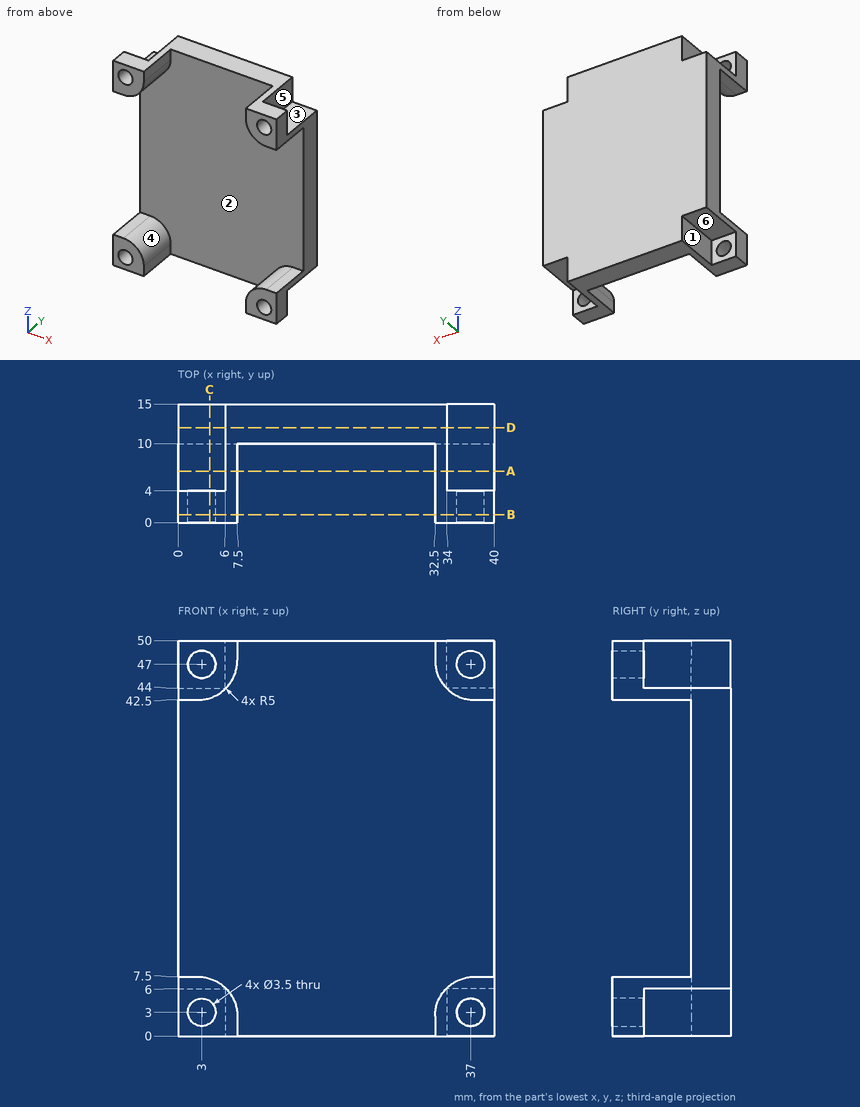
Print and shaded views of the part. All mm, measured from the part's lowest x, y and z. A direction names the side the tool comes from. Give positions to 0.01 mm unless a question says otherwise; leave off trailing zeros. Write each loop counter-clockwise with the first axis right and the second up, starting at its lowest first coordinate (ties: lowest second). Pieces come first, ordered by that corner, then holes. Notation, with made-up numbers: (62.25, 68.5) - (71.25, 68.5) arc R6 ccw to (71.25, 79.5) - close; hole circle Ø7 at (-5, 28.5). An arc over 180 degrees is marked (long way). One line per question, with ' | ' between items. Start each with the question number.
(1) Slice it at D-D on y = 12. Write the cut outline in (x, z).
(2) Wall check: line 1 along X through (y, z) = (2.5, 47); line 2 along Z through (x, y) = (37, 0.8); line 3 along Y through (x, z) = (14.5, 39.5). Give the ranges that are in metal, low to high. Write a range as from..to.
(3) Slice it at C-C on x = 4. Write the cut outline in (y, z).
(4) 3-axis set-ups, long thin cutter, end or side, ignore diameter. For the marked faces 1, 2 and 3: which of +Z, -Z, +X, -X, +Y, -Y reach the whole face in a straight line?
(5) Pin check, flat tips, straight feed: P1, Ø0.8, axis at y = 5.5, z = 0.5, coming from the -X side; P2, Ø0.8, axis at x = 2, y = 5.5, coming from the +Z side; P3, Ø4, axis at y = 7.5, z = 22, coming from the +X side; P4, Ø1.8, axis at x = 3, z = 48.5, coming from the +Y side. Stop position of each tip, or through.
(6) Two-plate mould, pull along Z, no slides. Class the marked faces 4, 5 and 6: +Z half, -Z half, draft (parallel to the pull), parting line (faces both ways), or undercut.
(7) Slice it at B-B on y = 1. Write the cut outline in (x, z).
(8) Slice it at A-A on y = 6.5. Write the cut outline in (x, z), plus the area to 3 significant figures.
Results below:
1) outline: (0, 6) - (6, 6) - (6, 0) - (34, 0) - (34, 6) - (40, 6) - (40, 44) - (34, 44) - (34, 50) - (6, 50) - (6, 44) - (0, 44) - close
2) line 1: 0..1.25, 4.75..7.47, 32.53..35.25, 38.75..40 | line 2: 0..1.25, 4.75..7.47, 42.53..45.25, 48.75..50 | line 3: 10..15
3) outline: (0, 0) - (4, 0) - (4, 1.56) - (0, 1.56) - close; (0, 4.44) - (4, 4.44) - (4, 6) - (15, 6) - (15, 44) - (4, 44) - (4, 45.56) - (0, 45.56) - (0, 42.73) - (10, 42.73) - (10, 7.27) - (0, 7.27) - close; (0, 48.44) - (4, 48.44) - (4, 50) - (0, 50) - close
4) face 1: -Z, -X, +Y | face 2: -Y | face 3: +Z, +X, +Y
5) P1: x = 6 | P2: z = 44 | P3: through | P4: y = 4
6) face 4: undercut | face 5: draft | face 6: -Z half
7) outline: (0, 0) - (7.5, 0) - (7.5, 2.5) arc R5 ccw to (2.5, 7.5) - (0, 7.5) - close; (0, 42.5) - (2.5, 42.5) arc R5 ccw to (7.5, 47.5) - (7.5, 50) - (0, 50) - close; (32.5, 0) - (40, 0) - (40, 7.5) - (37.5, 7.5) arc R5 ccw to (32.5, 2.5) - close; (32.5, 47.5) arc R5 ccw to (37.5, 42.5) - (40, 42.5) - (40, 50) - (32.5, 50) - close; hole circle Ø3.5 at (3, 3); hole circle Ø3.5 at (3, 47); hole circle Ø3.5 at (37, 3); hole circle Ø3.5 at (37, 47)
8) outline: (0, 6) - (6, 6) - (6, 0) - (7.5, 0) - (7.5, 2.5) arc R5 ccw to (2.5, 7.5) - (0, 7.5) - close; (0, 42.5) - (2.5, 42.5) arc R5 ccw to (7.5, 47.5) - (7.5, 50) - (6, 50) - (6, 44) - (0, 44) - close; (32.5, 0) - (34, 0) - (34, 6) - (40, 6) - (40, 7.5) - (37.5, 7.5) arc R5 ccw to (32.5, 2.5) - close; (32.5, 47.5) arc R5 ccw to (37.5, 42.5) - (40, 42.5) - (40, 44) - (34, 44) - (34, 50) - (32.5, 50) - close | area: 59.5 mm^2
